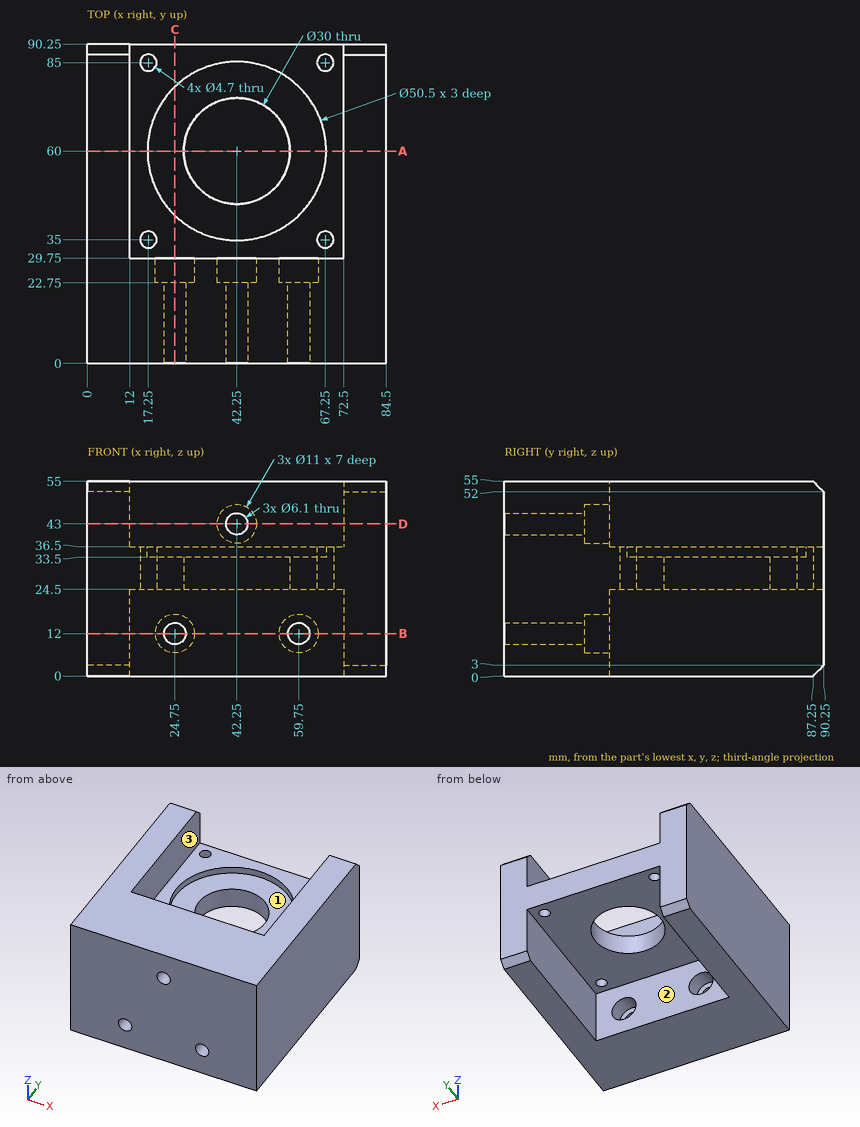
Print and shaded views of the part. All mm, measured from the part's lowest x, y and z. A direction names the side the tool comes from. Round coordinates to 2 decimals unless told otherwise and drop trailing zeros. Loops run counter-clockwise (first coordinate to the right, second up) from the corner with the lowest first, then second, coordinate; pieces in that order, holes last. Notation, with made-up numbers: (-3.5, 14) -> (44.5, 14) arc R20 cw to (44.5, 44) -> close; hole circle Ø7 at (-18.5, -6.75). An arc over 180 degrees is marked (long way). Use CSV: the item, a comma, the result in double quotes. Start each with the question number.
1) Cut at A-A, the plane y = 60. Write the cut outline in (x, z).
2) Wall check: L1, parallel to X at y = 6, z = 12; L2, parallel to Y at x = 17, z = 32; L3, parallel to X at y = 85.5, z = 18. Give the ranges that are in metal, low to high. Write a range as [from, to].
3) Drop flat-ended pins along their axis: P1, Ø9, axis at y = 63, z = 44.5, coming from the -X side; P2, Ø25, axis at x = 41, y = 48.5, coming from the +Z side; P3, Ø18, axis at x = 40, y = 74, coming from the -Z side; P4, Ø5.5, axis at x = 24, z = 12, coming from the +Y side. Give the stop position or say it passes through.
4) Cut at B-B, the plane z = 12. Write the cut outline in (x, y).
5) Which spindle directions (+Z, -Z, +X, -X, +Y, -Y) get a long thin tool onto all of the face, cutting with end or side? Do the marked faces 1, 2 and 3. Say none if no direction does.
6) Cut at C-C, the plane x = 24.75. Write the cut outline in (y, z).
7) Cut at D-D, the plane z = 43. Write the cut outline in (x, y), plus the area to 3 significant figures.
Determined:
1,outline,"(0, 0) -> (12, 0) -> (12, 24.5) -> (27.25, 24.5) -> (27.25, 33.5) -> (17, 33.5) -> (17, 36.5) -> (12, 36.5) -> (12, 55) -> (0, 55) -> close; (57.25, 24.5) -> (72.5, 24.5) -> (72.5, 0) -> (84.5, 0) -> (84.5, 55) -> (72.5, 55) -> (72.5, 36.5) -> (67.5, 36.5) -> (67.5, 33.5) -> (57.25, 33.5) -> close"
2,L1,"x = [0, 21.7], [27.8, 56.7], [62.8, 84.5]"
2,L2,"y = [0, 32.66], [37.34, 82.66], [87.34, 90.25]"
2,L3,"x = [0, 12], [72.5, 84.5]"
3,P1,"stops at x = 0"
3,P2,"stops at z = 33.5"
3,P3,"stops at z = 24.5"
3,P4,"stops at y = 22.75"
4,outline,"(0, 0) -> (21.7, 0) -> (21.7, 22.75) -> (19.25, 22.75) -> (19.25, 29.75) -> (12, 29.75) -> (12, 90.25) -> (0, 90.25) -> close; (27.8, 0) -> (56.7, 0) -> (56.7, 22.75) -> (54.25, 22.75) -> (54.25, 29.75) -> (30.25, 29.75) -> (30.25, 22.75) -> (27.8, 22.75) -> close; (62.8, 0) -> (84.5, 0) -> (84.5, 90.25) -> (72.5, 90.25) -> (72.5, 29.75) -> (65.25, 29.75) -> (65.25, 22.75) -> (62.8, 22.75) -> close"
5,face 1,"+Z"
5,face 2,"-Z, +Y"
5,face 3,"+Z, +Y"
6,outline,"(0, 0) -> (29.75, 0) -> (29.75, 6.5) -> (22.75, 6.5) -> (22.75, 8.95) -> (0, 8.95) -> close; (0, 15.05) -> (22.75, 15.05) -> (22.75, 17.5) -> (29.75, 17.5) -> (29.75, 24.5) -> (90.25, 24.5) -> (90.25, 36.5) -> (78.2, 36.5) -> (78.2, 33.5) -> (41.8, 33.5) -> (41.8, 36.5) -> (29.75, 36.5) -> (29.75, 55) -> (0, 55) -> close"
7,outline,"(0, 0) -> (39.2, 0) -> (39.2, 22.75) -> (36.75, 22.75) -> (36.75, 29.75) -> (12, 29.75) -> (12, 90.25) -> (0, 90.25) -> close; (45.3, 0) -> (84.5, 0) -> (84.5, 90.25) -> (72.5, 90.25) -> (72.5, 29.75) -> (47.75, 29.75) -> (47.75, 22.75) -> (45.3, 22.75) -> close"
7,area,"3,750 mm2"
